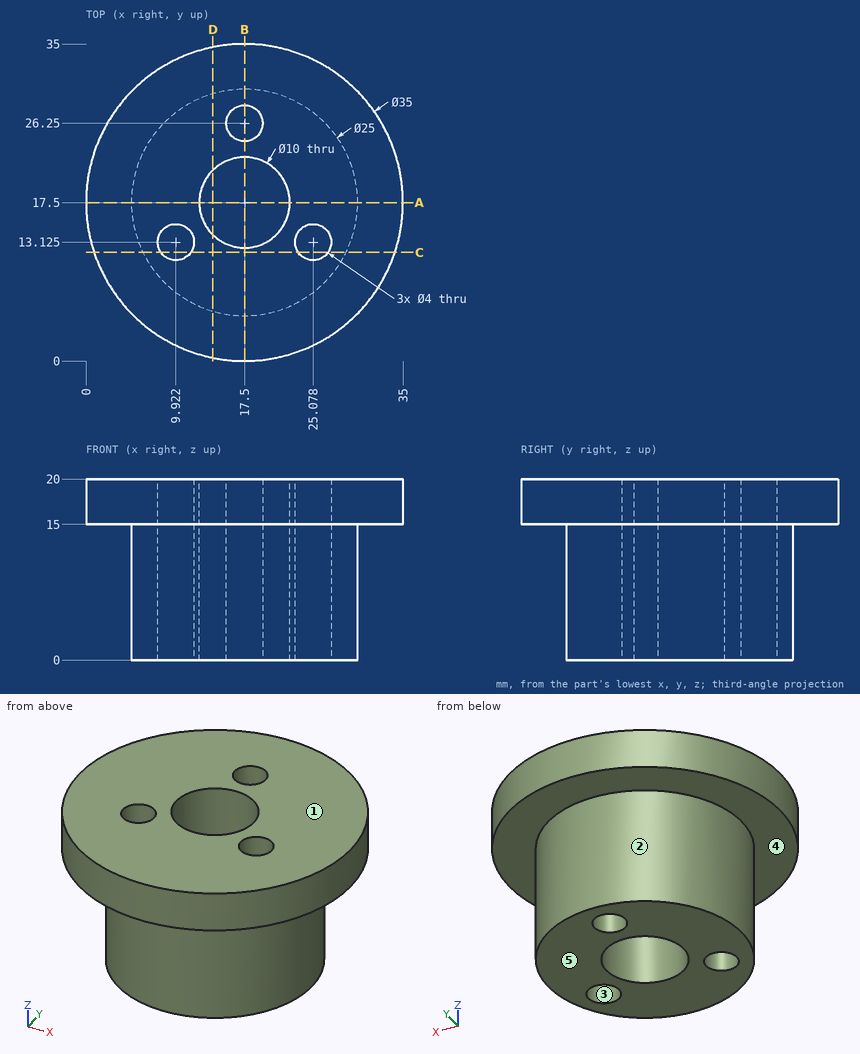
Job drawing, mm, ordinate dimensions from the low corner. One solid piece. A direction names the side the tool comes from. Give positions to 0.01 mm unless a question says otherwise; leave off trailing zeros. Order: outer loops, then holes, each group sorted by start corner. A loop starts at its lowest first (then second) coordinate and runs counter-clockwise, first axis right, second up. Notation, with made-up numbers: (14.25, -26.75) - (21.25, -26.75) arc R31 cw to (21.25, 12.25) - close; hole circle Ø5 at (35.5, 27). An arc over 180 degrees is marked (long way). Return JSON: item names as keys, results as strings.
1) 3-axis set-ups, long thin cutter, end or side, ignore diameter. For the marked faces 4 and 5: which of +Z, -Z, +X, -X, +Y, -Y reach the whole face in a straight line?
Geometry says:
{"face 4": "-Z", "face 5": "-Z, +X, -X, +Y, -Y"}
2) Cut at D-D, the plane x = 14. Give the cut face in (y, z), plus the area to 3 significant figures.
Geometry says:
{"outline": "(0.35, 15) - (5.5, 15) - (5.5, 0) - (13.93, 0) - (13.93, 20) - (0.35, 20) - close; (21.07, 0) - (29.5, 0) - (29.5, 15) - (34.65, 15) - (34.65, 20) - (21.07, 20) - close", "area": "389 mm²"}
3) Probe line 1 (Y direction, x = 17.5, z = 5); line 2 (Z direction, x = 7, y = 26); line 3 (X direction, y = 14.5, z = 10) (1 decimal). List the from-to ranges inside material, lowest first. Write a range as from..to.
Geometry says:
{"line 1": "5..12.5, 22.5..24.25, 28.25..30", "line 2": "15..20", "line 3": "5.4..8.5, 11.4..13.5, 21.5..23.6, 26.5..29.6"}
4) Pull direction X, two halves, no side cores. Call the marked faces 1, 2 and 3: pulls with the +X half, pulls with the -X half, needs draft (parallel to the pull), parting line crosses it, or undercut.
Geometry says:
{"face 1": "needs draft", "face 2": "parting line crosses it", "face 3": "undercut"}
5) Cut at C-C, the plane y = 12. Give the cut face in (x, z) (1 decimal).
Geometry says:
{"outline": "(0.9, 15) - (6.3, 15) - (6.3, 0) - (8.3, 0) - (8.3, 20) - (0.9, 20) - close; (11.6, 0) - (23.4, 0) - (23.4, 20) - (11.6, 20) - close; (26.7, 0) - (28.7, 0) - (28.7, 15) - (34.1, 15) - (34.1, 20) - (26.7, 20) - close"}
6) Cut at B-B, the plane x = 17.5. Give the cut face in (y, z), plus the area to 3 significant figures.
Geometry says:
{"outline": "(0, 15) - (5, 15) - (5, 0) - (12.5, 0) - (12.5, 20) - (0, 20) - close; (22.5, 0) - (24.25, 0) - (24.25, 20) - (22.5, 20) - close; (28.25, 0) - (30, 0) - (30, 15) - (35, 15) - (35, 20) - (28.25, 20) - close", "area": "270 mm²"}
7) Flat gauge pins, fed straight in: P1, Ø2.5, axis at x = 17.5, y = 26.25, coming from the -Z side; P2, Ø1.5, axis at y = 11, z = 5, coming from the +X side; P3, Ø5, axis at x = 12.5, z = 17, coming from the -Y side; P4, Ø2, axis at x = 5.5, y = 6, coming from the -Z side. Where does each tip first touch, or does it go through?
Geometry says:
{"P1": "through", "P2": "x = 28.6", "P3": "y = 0.18", "P4": "z = 15"}
8) Cut at A-A, the plane y = 17.5. Give the cut face in (x, z), plus the area to 3 significant figures.
Geometry says:
{"outline": "(0, 15) - (5, 15) - (5, 0) - (12.5, 0) - (12.5, 20) - (0, 20) - close; (22.5, 0) - (30, 0) - (30, 15) - (35, 15) - (35, 20) - (22.5, 20) - close", "area": "350 mm²"}
